Verification items for this drawing (mm, ordinates from the low corner). Round coordinates to 2 decimals unless told otherwise and drop trailing zeros. Loops run counter-clockwise (first coordinate to the right, second up) from the corner with the lowest first, then second, coordinate; pieces in that order, holes last. Notation, with made-up numbers: (-19, 51.5) -> (22, 51.5) arc R36 cw to (22, 87.5) -> close; hole circle Ø4 at (47.25, 7). An arc over 180 degrees is marked (long way). One line per item, written item: value. Start each with the question number.
1. Go/stop test with flat-tipped pins: pin 1 (0.9 mm diameter, centred on x = 289, z = 1, fed in from -Y); pin 2 (1.5 mm diameter, centred on y = 64, z = 2, fed in from +X). Record where each tip stops, or that it passes through.
2. Cross-section at B-B on y = 99. Record the cut outline in (x, z).
3. Cross-section at A-A on z = 1.5. Record the cut outline in (x, y).
4. Material ranges on L1, parallel to X at y = 104.5, z = 0.9, recorded low to high.
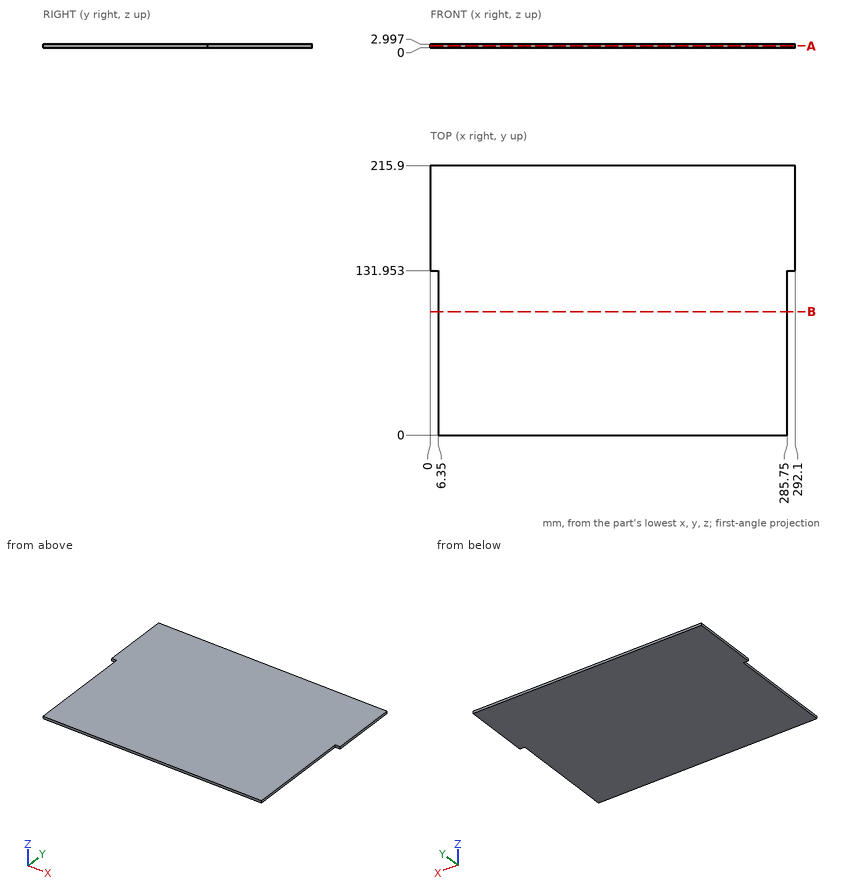
Taken from the geometry:
1. pin 1: stops at y = 131.95
1. pin 2: stops at x = 285.75
2. outline: (6.35, 0) -> (285.75, 0) -> (285.75, 3) -> (6.35, 3) -> close
3. outline: (0, 131.95) -> (6.35, 131.95) -> (6.35, 0) -> (285.75, 0) -> (285.75, 131.95) -> (292.1, 131.95) -> (292.1, 215.9) -> (0, 215.9) -> close
4. L1: x = 6.35 to 285.75
